```python
from build123d import *

# Parameters (mm, degrees)
EXTRUDE_1_DEPTH     = 1.8
EXTRUDE_2_DEPTH     = 3.8
FILLET_1_R          = 2
SKETCH_5_R          = 4
CUT_EXTRUDE_1_DEPTH = 4
SKETCH_6_R          = 6
CUT_EXTRUDE_2_DEPTH = 1.5


with BuildPart() as part:
    # Эскиз1 → Бобышка-Вытянуть1 (new body)
    with BuildSketch(Plane(origin=(0, 0, 0), x_dir=(1, 0, 0), z_dir=(0, 1, 0))):
        with BuildLine():
            Line((-15, 43.349382745), (-16.35, 28))
            Line((-16.35, 28), (-16.35, 4))
            ThreePointArc((-16.35, 4), (-16.203553391, 3.646446609), (-15.85, 3.5))
            Line((-15.85, 3.5), (-15.35, 3.5))
            Line((-15.35, 3.5), (-15.35, -3.5))
            Line((-15.35, -3.5), (-15.85, -3.5))
            ThreePointArc((-15.85, -3.5), (-16.203553391, -3.646446609), (-16.35, -4))
            Line((-16.35, -4), (-16.35, -28))
            Line((-16.35, -28), (-15, -43.35061617))
            Line((-15, -43.35061617), (0, -43.784698928))
            Line((0, -43.784698928), (15, -43.35061617))
            Line((15, -43.35061617), (16.35, -28))
            Line((16.35, -28), (16.35, 28))
            Line((16.35, 28), (15, 43.349382745))
            Line((15, 43.349382745), (0, 43.915301072))
            Line((0, 43.915301072), (-15, 43.349382745))
        make_face()
    extrude(amount=EXTRUDE_1_DEPTH)

    # Эскиз4 → Бобышка-Вытянуть2 (add)
    with BuildSketch(Plane(origin=(0, 0, 0), x_dir=(1, 0, 0), z_dir=(0, 1, 0))):
        Polygon((-13.3, 40.75), (-13.3, -40.75), (0, -41.25), (13.3, -40.75), (13.3, 40.75), (0, 41.25), align=None)
    extrude(amount=EXTRUDE_2_DEPTH)

    # Скругление1
    fillet_1_edges = [part.edges().sort_by_distance(p)[0] for p in [
        (-15, 0.9, -43.349382745),
        (15, 0.9, -43.349382745),
        (15, 0.9, 43.35061617),
        (-15, 0.9, 43.35061617),
    ]]
    fillet(fillet_1_edges, radius=FILLET_1_R)

    # Эскиз5 → Вырез-Вытянуть1 (cut)
    with BuildSketch(Plane(origin=(0, 3.8, 0), x_dir=(-1, 0, 0), z_dir=(0, 1, 0))):
        with Locations(Location((-0.3, 0, 0), (0, 0, 90))):
            Circle(SKETCH_5_R)
    extrude(amount=-CUT_EXTRUDE_1_DEPTH, mode=Mode.SUBTRACT)

    # Эскиз6 → Вырез-Вытянуть2 (cut)
    with BuildSketch(Plane(origin=(0, 3.8, 0), x_dir=(1, 0, 0), z_dir=(0, 1, 0))):
        with Locations(Location((0.3, 0, 0), (0, 0, 270))):
            Circle(SKETCH_6_R)
    extrude(amount=-CUT_EXTRUDE_2_DEPTH, mode=Mode.SUBTRACT)


solid = part.part
```
Part model, mm, in its own coordinate system. A direction names the side the tool comes from. Round coordinates to 2 decimals unless told otherwise and drop trailing zeros. Order: outer loops, then holes, each group sorted by start corner. A loop starts at its lowest first (then second) coordinate and runs counter-clockwise, first axis right, second up. Notation, with made-up numbers: M -28.75,29.25 L 30.25,29.25 A15 cw 30.25,54.25 Z; hole C 62,82 d1. An arc over 180 degrees is marked long. Answer in a Markdown table with one row per item. Add a question column.
Q1. Mould opens along Z. For faces 5 (the face through (-6, 3.8, -1)), 6 (the face through (-2.1, 1.2, -3.2)), 7 (the face through (14.526, 0.913, -42.88)) say: +Z half, -Z half, draft (parallel to the pull), parting line (faces both ways), or undercut.
Q2. Cut at C-C on z = 23. Give the cut face in (x, y), and give its area (3 significant figures).
Q3. 3-axis set-ups, long thin cutter, end or side, ignore diameter. For faces 1 (the face through (-6.7, 2.8, 41)), 2 (the face through (6.6, 2.8, 41)), 3 (the face through (-6.6, 2.8, -41)), 4 (the face through (-1, 2.3, 4)): which of +Z, -Z, +X, -X, +Y, -Y reach the whole face in a straight line?
Q4. Pin check, flat tips, straight feed: pin 1 (1 mm diameter, centred on x = 11, y = 0.5, fed in from +Z); pin 2 (10.5 mm diameter, centred on x = 0.3, z = 0, fed in from +Y); pin 3 (0.6 mm diameter, centred on y = 3, z = -13.5, fed in from +X). Stop position of each tip, or through.
Q5. Cut at A-A on y = 3.05. Give the cut face in (x, z), and give its area (3 significant figures).
Q6. Cut at B-B on z = 0. Give the cut face in (x, y).
Q7. Cut at D-D on x = 10. Give the cut face in (y, z), and give its area (3 significant figures).
Q8. Wall check: L1, parallel to X at y = 0.7, z = 0; L2, parallel to X at y = 3.1, z = 0; L3, parallel to Y at x = 13.5, z = -19.5. Give the ranges that are in metal, low to high. Write a range as from..to.
Established:
| question | item | result |
|---|---|---|
| 1 | face 5 | draft |
| 1 | face 6 | undercut |
| 1 | face 7 | -Z half |
| 2 | outline | M -16.35,0 L 16.35,0 L 16.35,1.8 L 13.3,1.8 L 13.3,3.8 L -13.3,3.8 L -13.3,1.8 L -16.35,1.8 Z |
| 2 | area | 112 mm2 |
| 3 | face 1 | +Z, -X, +Y |
| 3 | face 2 | +Z, +X, +Y |
| 3 | face 3 | -Z, -X, +Y |
| 3 | face 4 | +Y |
| 4 | pin 1 | stops at z = 43.48 |
| 4 | pin 2 | stops at y = 2.3 |
| 4 | pin 3 | stops at x = 13.3 |
| 5 | outline | M -13.3,-40.75 L 0,-41.25 L 13.3,-40.75 L 13.3,40.75 L 0,41.25 L -13.3,40.75 Z; hole C 0.3,0 d12 |
| 5 | area | 2,070 mm2 |
| 6 | outline | M -15.35,0 L -3.7,0 L -3.7,2.3 L -5.7,2.3 L -5.7,3.8 L -13.3,3.8 L -13.3,1.8 L -15.35,1.8 Z; M 4.3,0 L 16.35,0 L 16.35,1.8 L 13.3,1.8 L 13.3,3.8 L 6.3,3.8 L 6.3,2.3 L 4.3,2.3 Z |
| 7 | outline | M 0,-43.54 L 1.8,-43.54 L 1.8,-40.87 L 3.8,-40.87 L 3.8,40.87 L 1.8,40.87 L 1.8,43.5 L 0,43.5 Z |
| 7 | area | 320 mm2 |
| 8 | L1 | x = -15.35..-3.7, 4.3..16.35 |
| 8 | L2 | x = -13.3..-5.7, 6.3..13.3 |
| 8 | L3 | y = 0..1.8 |
